from build123d import *

# Parameters (mm, degrees)
BOSS_EXTRU_2_DEPTH = 10
CONG_2_R           = 5
COQUE3_T           = 3


with BuildPart() as part:
    # Esquisse1 → Boss.-Extru.2 (new body)
    with BuildSketch(Plane.XY):
        Polygon((-15, 0), (15, 0), (9.5, 33.5), (-9.5, 33.5), align=None)
    extrude(amount=BOSS_EXTRU_2_DEPTH)

    # Congé2
    cong_2_edges = [part.edges().sort_by_distance(p)[0] for p in [
        (15, 0, 5),
        (-15, 0, 5),
        (-9.5, 33.5, 5),
        (9.5, 33.5, 5),
    ]]
    fillet(cong_2_edges, radius=CONG_2_R)

    # Coque3
    coque3_openings = [part.faces().sort_by_distance(p)[0] for p in [
        (0, 15.617025891, 0),
        (0, 15.617025891, 10),
    ]]
    offset(amount=COQUE3_T, openings=coque3_openings, kind=Kind.INTERSECTION)


solid = part.part
Design review of the part built by this model. Coordinates are the model's own, in mm. A direction names the side the tool comes from. Round coordinates to 2 decimals unless told otherwise and drop trailing zeros. Loops run counter-clockwise (first coordinate to the right, second up) from the corner with the lowest first, then second, coordinate; pieces in that order, holes last. Notation, with made-up numbers: (52.25, 79.5) -> (97.25, 79.5) arc R17 cw to (97.25, 105.5) -> close; hole circle Ø7 at (-20.5, -35.75). An arc over 180 degrees is marked (long way). Use one line per item in the form item = value. Start each with the question number.
Q1. We need section B-B on x = -2.5. Give the boundary of the cut face in (y, z), then the cut area to 3 significant figures.
Q2. Draft analysis for pull direction Y (two halves, no side actions). For faces 1 (the face through (-12.884, 1.718, 5.07)), 2 (the face through (-13, 14, 0)), 3 (the face through (15.1, 17.9, 4.9)), state which applies: +Y half, -Y half, draft (parallel to the pull), parting line (faces both ways), or undercut.
Q3. We need section A-A on z = 9.25. Give the boundary of the cut face in (x, y), then the cut area to 3 significant figures.
Q4. Wall thickness on line 1 along Y through (x, z) = (3.5, 3); line 2 along X through (y, z) = (22, 4.25); line 3 along X through (y, z) = (23, 4.25): over which ranges is each line inside the solid? List them lowest first. Write a range as [from, to].
Q5. We need section C-C on y = 31. Give the boundary of the cut face in (x, z), then the cut area to 3 significant figures.
Q6. Machinability: for faces 4 (the face through (-10.37, 34.65, 5.07)), 5 (the face through (0, 0, 5)), which of the approach directions +Z, -Z, +X, -X, +Y, -Y give a long, thin tool a straight path to every point of the face, cutting with its end or side? Answer none if there is none.
Q7. For pin 1 Ø1 at (x, y) = (11, 10.5) entering from -Z, flat-tipped, find the tip position at first contact; note if it passes through.
Calculated:
q1.outline = (-3, 0) -> (0, 0) -> (0, 10) -> (-3, 10) -> close; (33.5, 0) -> (36.5, 0) -> (36.5, 10) -> (33.5, 10) -> close
q1.area = 60.0 mm²
q2.face_1 = undercut
q2.face_2 = draft
q2.face_3 = +Y half
q3.outline = (-17.01, 6.3) arc R8 ccw to (-9.11, -3) -> (9.11, -3) arc R8 ccw to (17.01, 6.3) -> (13.15, 29.8) arc R8 ccw to (5.25, 36.5) -> (-5.25, 36.5) arc R8 ccw to (-13.15, 29.8) -> close; hole (-14.05, 5.81) arc R5 ccw to (-9.11, 0) -> (9.11, 0) arc R5 ccw to (14.05, 5.81) -> (10.19, 29.31) arc R5 ccw to (5.25, 33.5) -> (-5.25, 33.5) arc R5 ccw to (-10.19, 29.31) -> close
q3.area = 352 mm²
q4.line_1 = [-3, 0], [33.5, 36.5]
q4.line_2 = [-14.43, -11.39], [11.39, 14.43]
q4.line_3 = [-14.26, -11.22], [11.22, 14.26]
q5.outline = (-12.85, 0) -> (-9.58, 0) -> (-9.58, 10) -> (-12.85, 10) -> close; (9.58, 0) -> (12.85, 0) -> (12.85, 10) -> (9.58, 10) -> close
q5.area = 65.4 mm²
q6.face_4 = +Z, -Z, -X, +Y
q6.face_5 = +Z, -Z
q7.pin_1 = through
